Could you check a few things on this drawing? It's one solid part, dimensions in mm from its lowest x, y, z. A direction names the side the tool comes from. Round coordinates to 2 decimals unless told otherwise and drop trailing zeros. Write each loop counter-clockwise with the first axis right and the second up, starting at its lowest first coordinate (ties: lowest second). Pieces come first, ordered by that corner, then holes. Notation, with made-up numbers: (-36, 32.5) - (13, 32.5) arc R15 cw to (13, 60.5) - close; hole circle Ø2 at (21, 7.5). An arc over 180 degrees is marked (long way). Write item = value, one per line. Start each with the question number.
Item 1: If I drill on line 1 along X through (y, z) = (1, 5); line 2 along Y through (x, z) = (5.25, 0.75); line 3 along Y through (x, z) = (16, 8), over which ranges is the centre line in solid material (lowest first)? Write a range as [from, to].
Item 2: Thinking about a two-plate mould opening in Z: for the marked faces 1, 2 and 3, which applies, pulls with the +Z half, pulls with the -Z half, needs draft (parallel to the pull), parting line crosses it, or undercut?
Item 3: If we section it at D-D (z = 8): Please give me the cut outline in (x, y), and give its area (3 significant figures).
Item 4: Which directions (+Z, -Z, +X, -X, +Y, -Y) give clear straight access to the entire face, cutting with the end or side of a thin tool? Please do the marked faces 4, 5, 6 and 7.
Item 5: If we section it at C-C (y = 3.25): Please give me the cut outline in (x, z).
Item 6: If we section it at A-A (x = 12): Please give me the cut outline in (y, z).
Item 7: For P1, Ø1.8, axis at y = 3.5, z = 11.5, coming from the +X side; P2, Ø1.6, axis at y = 1, z = 13, coming from the -X side; P3, Ø0.8, axis at x = 7.5, y = 3, coming from the +Z side, each with a flat end and sliding along its axis, tell me the tip position at first contact or that it passes through.
Item 8: If we section it at B-B (z = 5.5): Please give me the cut outline in (x, y).
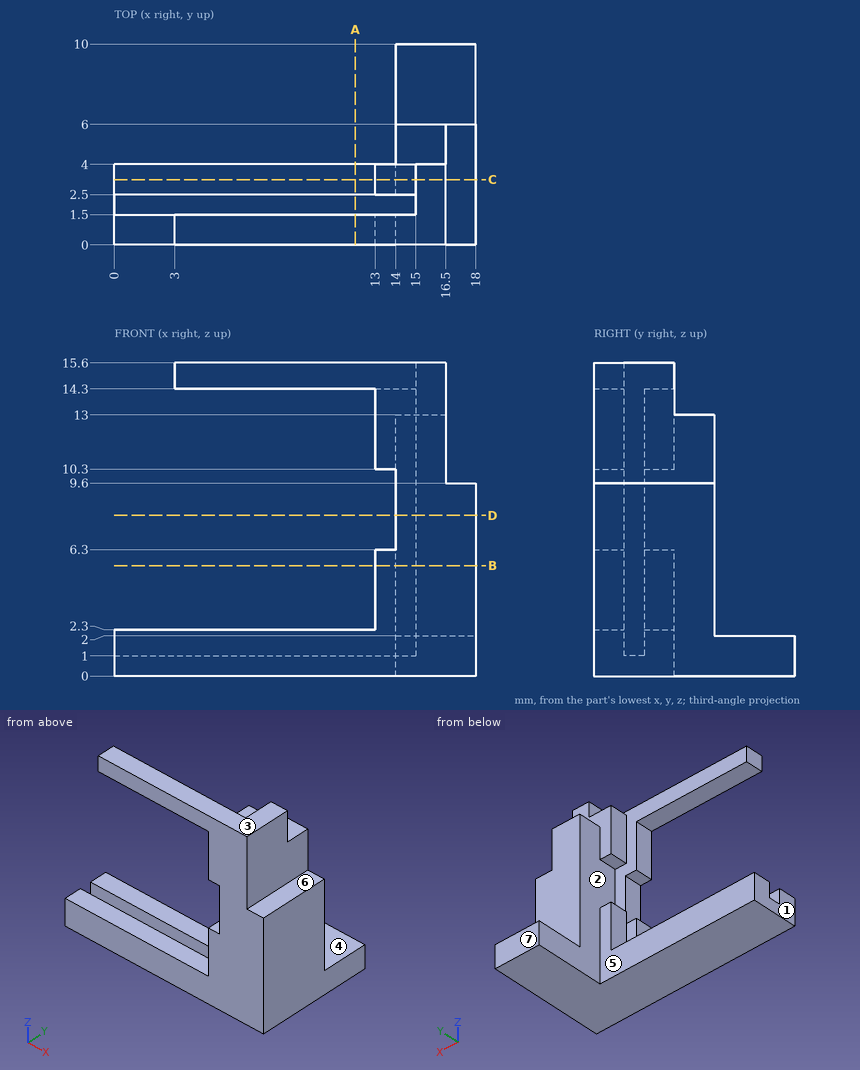
Reply:
q1.line_1 = [13, 18]
q1.line_2 = [0, 4]
q1.line_3 = [0, 6]
q2.face_1 = needs draft
q2.face_2 = undercut
q2.face_3 = pulls with the +Z half
q3.outline = (14, 0) - (18, 0) - (18, 6) - (14, 6) - (14, 2.5) - (15, 2.5) - (15, 1.5) - (14, 1.5) - close
q3.area = 23.0 mm2
q4.face_4 = +Z, +X, -X, +Y
q4.face_5 = +Z, -Z, -X, +Y
q4.face_6 = +Z, +X, +Y, -Y
q4.face_7 = +Z, -Z, +X, -X, +Y
q5.outline = (0, 0) - (18, 0) - (18, 9.6) - (16.5, 9.6) - (16.5, 15.6) - (15, 15.6) - (15, 14.3) - (13, 14.3) - (13, 10.3) - (14, 10.3) - (14, 6.3) - (13, 6.3) - (13, 2.3) - (0, 2.3) - close
q6.outline = (0, 0) - (4, 0) - (4, 2.3) - (2.5, 2.3) - (2.5, 1) - (1.5, 1) - (1.5, 2.3) - (0, 2.3) - close; (0, 14.3) - (1.5, 14.3) - (1.5, 15.6) - (0, 15.6) - close
q7.P1 = 16.5
q7.P2 = 13
q7.P3 = 2.3
q8.outline = (13, 0) - (18, 0) - (18, 6) - (14, 6) - (14, 4) - (13, 4) - (13, 2.5) - (15, 2.5) - (15, 1.5) - (13, 1.5) - close
